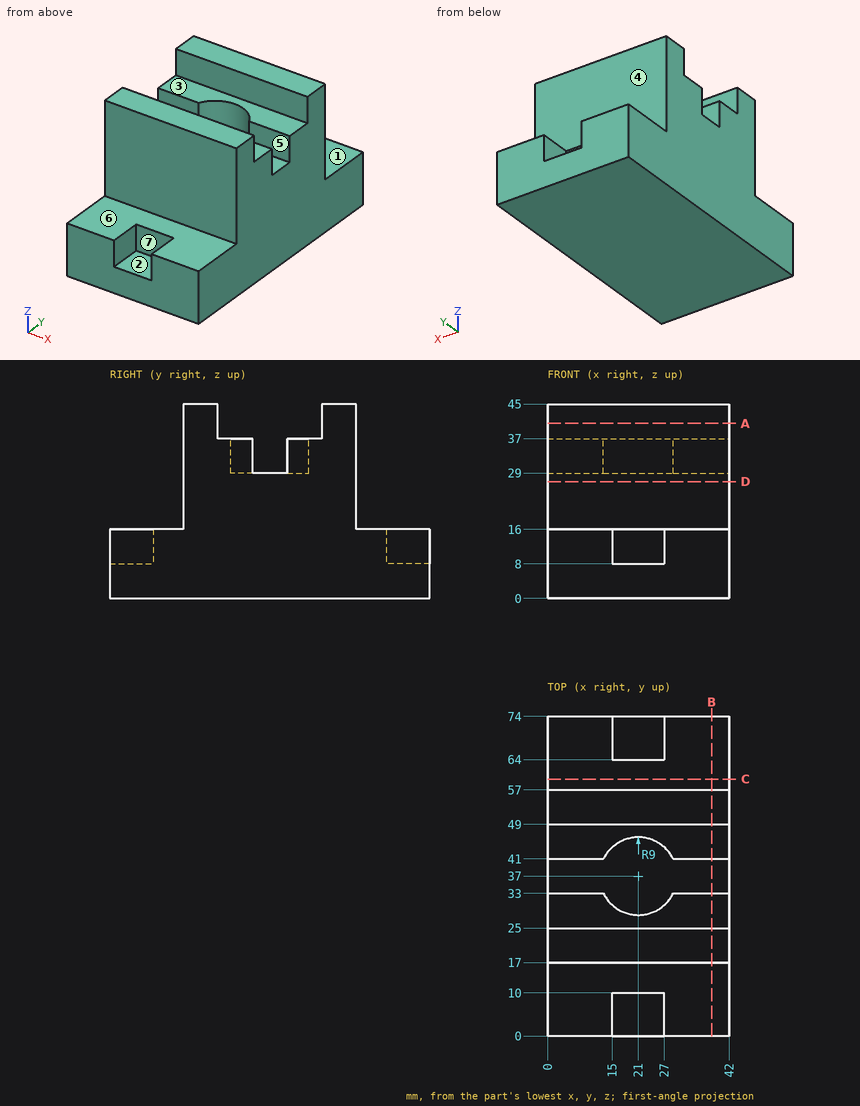
Source: three-view drawing plus pictorial views. Frame: mm from the lowest corner of the part. A direction names the side the tool comes from. Round coordinates to 2 decimals unless told otherwise and drop trailing zeros. Loops run counter-clockwise (first coordinate to the right, second up) from the corner with the lowest first, then second, coordinate; pieces in that order, holes last.
Item 1: Section A-A, the plane z = 40.5. Output: boundary loops of the cut face in (x, y).
Checked values:
outline: (0, 17) - (42, 17) - (42, 25) - (0, 25) - close; (0, 49) - (42, 49) - (42, 57) - (0, 57) - close
Item 2: Section C-C, the plane y = 59.5. Output: boundary loops of the cut face in (x, z).
Checked values:
outline: (0, 0) - (42, 0) - (42, 16) - (0, 16) - close
Item 3: Section D-D, the plane z = 27. Output: boundary loops of the cut face in (x, y).
Checked values:
outline: (0, 17) - (42, 17) - (42, 57) - (0, 57) - close
Item 4: Reachability of the marked faces 1, 2 and 3 from +Z, -Z, +X, -X, +Y, -Y: full face, straight path, thin tool, end or side. Return the list, or none.
Checked values:
face 1: +Z, +X, -X, +Y
face 2: +Z, -Y
face 3: +Z, +X, -X
Item 5: Section B-B, the plane x = 38. Output: boundary loops of the cut face in (y, z), plus the area to 3 significant figures.
Checked values:
outline: (0, 0) - (74, 0) - (74, 16) - (57, 16) - (57, 45) - (49, 45) - (49, 37) - (41, 37) - (41, 29) - (33, 29) - (33, 37) - (25, 37) - (25, 45) - (17, 45) - (17, 16) - (0, 16) - close
area: 2,090 mm2
Item 6: Contact query for flat-ended pins moving along their axis: P1, Ø9, axis at x = 12.5, y = 28.5, coming from the +Z side; P2, Ø9, axis at x = 7.5, z = 33.5, coming from the +Y side; P3, Ø5, axis at x = 15, y = 42.5, coming from the +Z side; P4, Ø6.5, axis at x = 19, z = 11.5, coming from the +Y side. Output: stop coordinate, or through.
Checked values:
P1: stops at z = 45
P2: stops at y = 57
P3: stops at z = 37
P4: stops at y = 64
Item 7: Mould query, pull axis Y, two halves, no side actions, for the marked faces 4, 5, 6 and 7. Classes: released by +Y, released by -Y, zero draft, split by the parting line, or undercut.
Checked values:
face 4: released by +Y
face 5: undercut
face 6: zero draft
face 7: released by -Y
Item 8: Line query: L1, parallel to Y at x = 37.5, z = 35.5; L2, parallel to Y at x = 3, z = 41.5; L3, parallel to X at y = 65.5, z = 10.5. Output: solid intervals per line, ascending.
Checked values:
L1: y = 17 to 33, 41 to 57
L2: y = 17 to 25, 49 to 57
L3: x = 0 to 15, 27 to 42
